Autodesk Inventor part; units mm, degrees
ref_plane "YZ Plane" through (0, 0, 0) normal (1, 0, 0) x (0, 1, 0)
ref_plane "XZ Plane" through (0, 0, 0) normal (0, 1, 0) x (-1, 0, 0)
ref_plane "XY Plane" through (0, 0, 0) normal (0, 0, 1) x (1, 0, 0)
sketch "Sketch1" plane through (0, 0, 0) normal (0, 0, 1) x (1, 0, 0)
  line L0 (22, 110) -> (0, 110)
  line L1 (0, 110) -> (0, 58)
  line L2 (0, 58) -> (0, 0) construction
  line L3 (0, 0) -> (22, 0) construction
  line L4 (22, 110) -> (22, 58)
  line L5 (22, 58) -> (0, 58)
  line L6 (22, 58) -> (22, 0) construction
  dimension "d0" = 220
  dimension "d1" = 22
  dimension "d6" = 116
revolve "Revolution1" add sketch "Sketch1" angle 360 about axis through (0, 0, 0) along (1, 0, 0)
sketch "Sketch2" plane through (0, 0, 0) normal (-1, 0, 0) x (0, 0, 1)
  circle A0 centre (0, 0) radius 58
  circle A1 centre (0, 0) radius 90 construction
  line L0 (0, 90) -> (0, 0) construction
  circle A2 centre (0, 0) radius 110
  circle A3 centre (34.4415, 83.1492) radius 9
  line L1 (0, 0) -> (34.4415, 83.1492) construction
  dimension "d2" = 180
  dimension "d7" = 18
  dimension "d8" = 22.5
extrude "Extrusion1" cut sketch "Sketch2" against normal through all contours A3
pattern_circular "Circular Pattern1" count 8 over 360 about axis through (11, 0, 0) along (1, 0, 0) of "Extrusion1"
equation "\"d0\" = D"
equation "\"d1\" = C1"
equation "\"d6\" = B1"
equation "\"d2\" = K1"
equation "\"d7\" = L"
equation "\"C1\" = 22"
equation "\"D\" = 220"
equation "\"K1\" = 180"
equation "\"L\" = 18"
equation "\"B1\" = 116"
equation "\"NB\" = 1.2345"
equation "\"Size_Designation\" = 1.2345"
properties part number "ISO 7005-1 Plate Flange for Welding Type 01 Flat Face - ISO PN 16 DN100" material "Steel"
Could you check a few things on this model? Use its own coordinates, in mm. Round coordinates to 2 decimals unless told otherwise and drop trailing zeros. Loops run counter-clockwise (first coordinate to the right, second up) from the corner with the lowest first, then second, coordinate; pieces in that order, holes last. Notation, with made-up numbers: M 28,-15 L 79,-15 A26 cw 79,24 Z; hole C -36,0.25 d2. An arc over 180 degrees is marked long. Write item = value, one per line.
1. I want a section at A-A, the plane y = 0. Write out the boundary of the cut face in (x, z).
Results below:
outline = M 0,-110 L 22,-110 L 22,-58 L 0,-58 Z; M 0,58 L 22,58 L 22,110 L 0,110 Z
2. Will these pins go through, and if not, where does the flat tip stop? P1, Ø8, axis at x = 10, z = -81, coming from the +Y side; P2, Ø2, axis at x = 18, z = 23.5, coming from the +Y side; P3, Ø3, axis at x = 3, z = 12.5, coming from the -Y side.
Results below:
P1 = 78.56
P2 = 107.67
P3 = -109.45
3. I want a section at B-B, the plane z = 86. Write out the boundary of the cut face in (x, y).
Results below:
outline = M 0,-68.59 L 22,-68.59 L 22,-42.98 L 0,-42.98 Z; M 0,-25.9 L 22,-25.9 L 22,25.9 L 0,25.9 Z; M 0,42.98 L 22,42.98 L 22,68.59 L 0,68.59 Z
4. I want a section at D-D, the plane x = 4. Count the separate pieces of the cut face and the enclosed holes in it, and give its area (3 significant figures).
Results below:
separate_pieces = 1
enclosed_holes = 9
area = 25,400 mm²
5. Thinking about a two-plate mould opening in Z: for faces 1 (the face through (22, 47, -47)), 2 (the face through (10.846, -23.846, 107.384)), 3 (the face through (10.85, 91.13, -30.28)), which applies, +Z half, -Z half, draft (parallel to the pull), parting line (faces both ways), or undercut?
Results below:
face_1 = draft
face_2 = parting line
face_3 = undercut
6. I need wall thicknesses on probe 1 along Y at (x, z) = (9, -2); probe 2 along Z at (x, y) = (7.25, 78.5); probe 3 along Y at (x, z) = (12, 75). Which ranges of each line are inside material? Lowest first, please.
Results below:
probe_1 = -109.98 to -57.97, 57.97 to 109.98
probe_2 = -77.06 to -42.15, -26.74 to 26.74, 42.15 to 77.06
probe_3 = -80.47 to -38.26, -30.62 to 30.62, 38.26 to 80.47
